from build123d import *

# Parameters (mm, degrees)
F0_W        = 80.775000155
F0_H        = 60.2360032499
F1_DEPTH    = 22
F2_T1_DEPTH = 106.175000155
F3_SIZE     = 10


# Not quite as in the source:
# - a fillet or chamfer that OpenCascade refuses, or shapes differently, is made with other operations: its cross-section is extruded or revolved along the edge and cut away or added


with BuildPart() as f1:
    # F0 (on Front) → F1 (new body)
    with BuildSketch(Plane.XZ):
        with Locations((0.7447451353, -30.1180016249)):
            Rectangle(F0_W, F0_H)
    extrude(amount=F1_DEPTH)

    # F2: fillet of radius 5.08 on 1 edges, made by hand

    # F2_s2 → F2_t1 (cut)
    with BuildSketch(Plane.YZ.offset(-52.3427549422)):
        with BuildLine():
            add(Edge.make_bspline(
                [(-16.92, -60.2360032499), (-22, -60.2360032499), (-22, -55.1560032499)],
                knots=[0, 0, 0, 1, 1, 1], degree=2, weights=[1, 1, 1]))
            Line((-22, -55.1560032499), (-22, -60.2360032499))
            Line((-22, -60.2360032499), (-16.92, -60.2360032499))
        make_face()
    extrude(amount=F2_T1_DEPTH, mode=Mode.SUBTRACT)

    # F3
    f3_edges = [f1.edges().sort_by_distance(p)[0] for p in [
        (0.744745, -22, 0),
    ]]
    chamfer(f3_edges, length=F3_SIZE)


solid = f1.part
Verification items for the finished model (mm, model axes). Give positions to 0.01 mm unless a question says otherwise; leave off trailing zeros. Loops run counter-clockwise (first coordinate to the right, second up) from the corner with the lowest first, then second, coordinate; pieces in that order, holes last.
1. Material ranges on probe 1 along Z at (x, y) = (32, -16.5); probe 2 along Z at (x, y) = (-36, -15.5), recorded low to high.
Derived:
probe 1: z = -60.24 to -4.5
probe 2: z = -60.24 to -3.5
2. Cross-section at A-A on z = -7. Record the cut outline in (x, y).
Derived:
outline: (-39.64, -19) - (41.13, -19) - (41.13, 0) - (-39.64, 0) - close
3. Go/stop test with a flat-tipped pin: P1, Ø1, axis at x = 22.5, y = -19.5, coming from the +Z side. Record where the tip stops, or that it passes through.
Derived:
P1: stops at z = -7
4. Cross-section at B-B on y = -15.5. Record the cut outline in (x, z).
Derived:
outline: (-39.64, -60.24) - (41.13, -60.24) - (41.13, -3.5) - (-39.64, -3.5) - close
